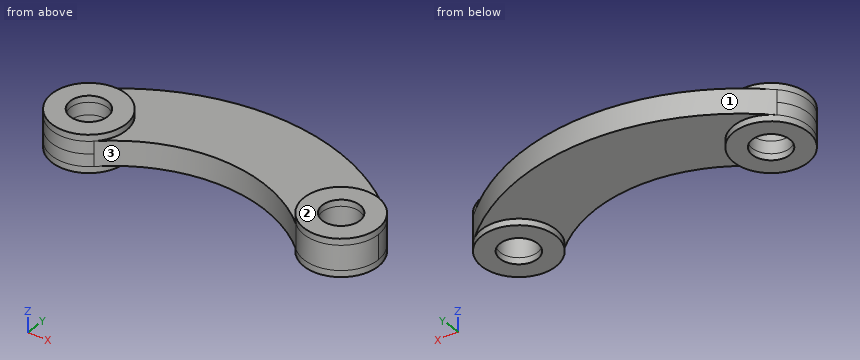
from build123d import *

# Parameters (mm, degrees)
SKETCH1_R           = 38
BOSS_EXTRUDE1_DEPTH = 25
SKETCH2_R           = 75
SKETCH2_R_2         = 38
BOSS_EXTRUDE2_DEPTH = 38


with BuildPart() as part:
    # Sketch1 → Boss-Extrude1 (new, symmetric)
    with BuildSketch(Plane.XY):
        with BuildLine():
            ThreePointArc((-51.549865229, 54.475787235), (-55.04414314, -50.942539257), (50.328947368, -55.605728633))
            ThreePointArc((50.328947368, -55.605728633), (255, 23.26430826), (459.671052632, -55.605728633))
            ThreePointArc((459.671052632, -55.605728633), (565.04414314, -50.942539257), (561.549865229, 54.475787235))
            ThreePointArc((561.549865229, 54.475787235), (255, 176.526439145), (-51.549865229, 54.475787235))
        make_face()
        Circle(SKETCH1_R, mode=Mode.SUBTRACT)
        with Locations((510, 0)):
            Circle(SKETCH1_R, mode=Mode.SUBTRACT)
    extrude(amount=BOSS_EXTRUDE1_DEPTH, both=True)

    # Sketch2 → Boss-Extrude2 (add, symmetric)
    # profile 1 of 2: a face of its own
    with BuildSketch(Plane.XY):
        Circle(SKETCH2_R)
        Circle(SKETCH2_R_2, mode=Mode.SUBTRACT)
    # profile 2 of 2: a face of its own
    with BuildSketch(Plane.XY):
        with Locations((510, 0)):
            Circle(SKETCH2_R)
        with Locations((510, 0)):
            Circle(SKETCH2_R_2, mode=Mode.SUBTRACT)
    extrude(amount=BOSS_EXTRUDE2_DEPTH, both=True)


solid = part.part
Can you work these out from the model? Positions are in its coordinate system, mm. Face numbers are marked on the shaded views. Give positions to 0.01 mm unless a question says otherwise; leave off trailing zeros. Order: outer loops, then holes, each group sorted by start corner. A loop starts at its lowest first (then second) coordinate and runs counter-clockwise, first axis right, second up. Notation, with made-up numbers: M 12.25,-3.5 L 63.25,-3.5 A30 cw 63.25,21.5 Z; hole C 17,-1 d6. An arc over 180 degrees is marked long. Use a Markdown table: item, result. Add a question column.
Item 1: Suppose I cut it at A-A (z = 13). List the corners of the cut face in (x, y) for me, then the cut area to 3 significant figures.
Item 2: We'd pull the mould along X, two halves only. Please class the marked faces 1, 2 and 3: +X half, -X half, draft (parallel to the pull), parting line (faces both ways), or undercut.
Item 3: Suppose I cut it at C-C (y = 134). List the corners of the cut face in (x, z) for me.
Item 4: Will these pins go through, and if not, where does the flat tip stop? pin 1 (10 mm diameter, centred on y = 131, z = 15.5, fed in from +X); pin 2 (10 mm diameter, centred on x = 382.5, z = -25, fed in from +Y); pin 3 (6 mm diameter, centred on x = 194, y = 113, fed in from +Z).
Item 5: Suppose I cut it at D-D (x = 137). List the corners of the cut face in (y, z) for me.
Item 6: If I drill on L1, parallel to Y at x = 510, z = -33; L2, parallel to Y at x = 30.5, z = -8.5; L3, parallel to Z at x = 327, y = 111.5, over which ranges is the centre line in solid material (lowest first)? Write a range as [from, to].
Item 7: Suppose I cut it at B-B (x = 519). List the corners of the cut face in (y, z) for me, then the cut area to 3 significant figures.
Answer sheet:
| question | item | result |
|---|---|---|
| 1 | outline | M -51.55,54.48 A75 ccw 50.33,-55.61 A305 cw 459.67,-55.61 A75 ccw 561.55,54.48 A446 ccw Z; hole C 0,0 d76; hole C 510,0 d76 |
| 1 | area | 93,900 mm² |
| 2 | face 1 | parting line |
| 2 | face 2 | draft |
| 2 | face 3 | undercut |
| 3 | outline | M 64.93,-25 L 445.07,-25 L 445.07,25 L 64.93,25 Z |
| 4 | pin 1 | stops at x = 461.2 |
| 4 | pin 2 | stops at y = 159.37 |
| 4 | pin 3 | stops at z = 25 |
| 5 | outline | M -0.49,-25 L 160.63,-25 L 160.63,25 L -0.49,25 Z |
| 6 | L1 | y = [-75, -38], [38, 75] |
| 6 | L2 | y = [-68.52, -22.67], [22.67, 115.9] |
| 6 | L3 | z = [-25, 25] |
| 7 | outline | M -74.46,-38 L -36.92,-38 L -36.92,38 L -74.46,38 Z; M 36.92,-38 L 74.46,-38 L 74.46,-25 L 90,-25 L 90,25 L 74.46,25 L 74.46,38 L 36.92,38 Z |
| 7 | area | 6,480 mm² |
